Here's the drawing with two shaded views (mm, measured from the low corner). I have some questions. Coordinates: 2 decimals unless noted, no trailing zeros. Loops run counter-clockwise (first coordinate to the right, second up) from the corner with the lowest first, then second, coordinate; pieces in that order, holes last.
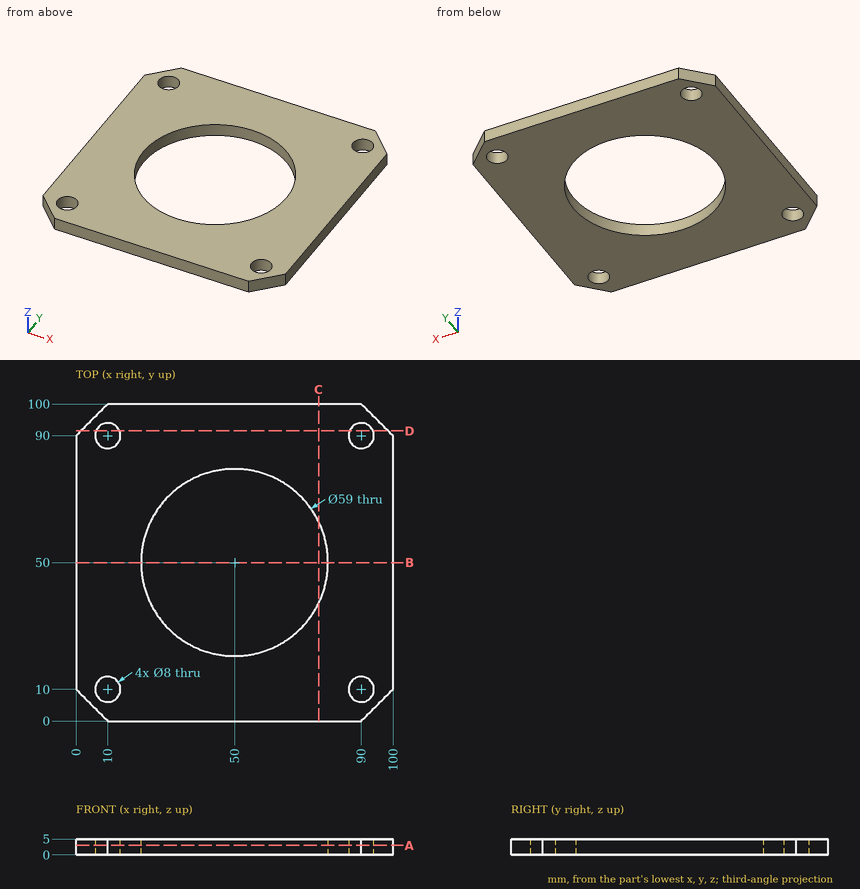
Q1. Will this pin go through, and if not, where does the flat tip stop? P1, Ø5, axis at x = 10, y = 90, coming from the +Z side.
Q2. Suppose I cut it at A-A on z = 3. Write out the boundary of the cut face in (x, y).
Q3. Suppose I cut it at B-B on y = 50. Write out the boundary of the cut face in (x, z), and give its area (3 significant figures).
Q4. Suppose I cut it at C-C on x = 76.5. Write out the boundary of the cut face in (y, z), and give its area (3 significant figures).
Q5. Suppose I cut it at D-D on y = 91.5. Write out the boundary of the cut face in (x, z), and give its area (3 significant figures).
Q6. Please list where these lines run through material, in increasing order: probe 1 along Y at (x, z) = (90, 3.05); probe 2 along X at (y, z) = (88.5, 4.1); probe 3 along Y at (x, z) = (13.5, 3.15).
Check values:
1. P1: passes through
2. outline: (0, 10) - (10, 0) - (90, 0) - (100, 10) - (100, 90) - (90, 100) - (10, 100) - (0, 90) - close; hole circle Ø8 at (10, 10); hole circle Ø8 at (10, 90); hole circle Ø59 at (50, 50); hole circle Ø8 at (90, 10); hole circle Ø8 at (90, 90)
3. outline: (0, 0) - (20.5, 0) - (20.5, 5) - (0, 5) - close; (79.5, 0) - (100, 0) - (100, 5) - (79.5, 5) - close
3. area: 205 mm2
4. outline: (0, 0) - (37.04, 0) - (37.04, 5) - (0, 5) - close; (62.96, 0) - (100, 0) - (100, 5) - (62.96, 5) - close
4. area: 370 mm2
5. outline: (1.5, 0) - (6.29, 0) - (6.29, 5) - (1.5, 5) - close; (13.71, 0) - (86.29, 0) - (86.29, 5) - (13.71, 5) - close; (93.71, 0) - (98.5, 0) - (98.5, 5) - (93.71, 5) - close
5. area: 411 mm2
6. probe 1: y = 0 to 6, 14 to 86, 94 to 100
6. probe 2: x = 0 to 6.29, 13.71 to 86.29, 93.71 to 100
6. probe 3: y = 0 to 8.06, 11.94 to 88.06, 91.94 to 100
